Design review of the part built by this model. Coordinates are the model's own, in mm. A direction names the side the tool comes from. Coordinates: 2 decimals unless noted, no trailing zeros. Loops run counter-clockwise (first coordinate to the right, second up) from the corner with the lowest first, then second, coordinate; pieces in that order, holes last. Notation, with made-up numbers: M 56,13 L 96,13 A15 cw 96,40 Z; hole C 31.5,70.5 d9. An arc over 180 degrees is marked long. Answer as CSV lines item,"result". Start each with the question number.
from build123d import *

# Parameters (mm, degrees)
F2_DEPTH  = 5
F3_W      = 14.7
F3_H      = 25
F4_DEPTH  = 7.7
F6_DEPTH  = 5
F8_DEPTH  = 70
F10_DEPTH = 5
F12_DEPTH = 50.001


with BuildPart() as f2:
    # F1 (on Top) → F2 (new body)
    with BuildSketch(Plane.XY):
        Polygon((0, 50), (0, 0), (17.65, 0), (17.65, 25), (32.35, 25), (32.35, 0), (50, 0), (50, 50), align=None)
    extrude(amount=F2_DEPTH)

    # F3 (on face) → F4 (join)
    with BuildSketch(Plane.XY.offset(5)):
        with Locations((25, 37.5)):
            Rectangle(F3_W, F3_H)
    extrude(amount=F4_DEPTH)

    # F5 (on face) → F6 (join)
    with BuildSketch(Plane.XY.offset(12.7)):
        Polygon((0, 50), (0, 0), (17.65, 0), (17.65, 25), (32.35, 25), (32.35, 0), (50, 0), (50, 50), align=None)
    extrude(amount=F6_DEPTH)

    # F7 (on face) → F8 (join)
    with BuildSketch(Plane.XY.offset(17.7)):
        with BuildLine():
            Line((32.35, 25), (32.35, 1.104865))
            ThreePointArc((32.35, 1.104865), (25, 50), (17.65, 1.104865))
            Line((17.65, 1.104865), (17.65, 25))
            Line((17.65, 25), (32.35, 25))
        make_face()
    extrude(amount=F8_DEPTH)

    # F9 (on face) → F10 (join)
    with BuildSketch(Plane.XY.offset(87.7)):
        with BuildLine():
            Line((0, 35), (0, 25))
            Line((0, 25), (50, 25))
            Line((50, 25), (50, 35))
            ThreePointArc((50, 35), (25, 60), (0, 35))
        make_face()
    extrude(amount=F10_DEPTH)

    # F11 (on Right) → F12 (cut, through all)
    with BuildSketch(Plane.YZ):
        Polygon((1.104865, 17.7), (25, 87.7), (1.104865, 87.7), align=None)
    extrude(amount=F12_DEPTH, mode=Mode.SUBTRACT)


solid = f2.part
Item 1: For pin 1 (3 mm diameter, centred on y = 23, z = 47, fed in from -X) (3 decimals); pin 2 (3 mm diameter, centred on y = 47, z = 25.5, fed in from -X); pin 3 (10 mm diameter, centred on x = 45, y = 29, fed in from -Z); pin 4 (2.5 mm diameter, centred on y = 38.5, z = 7, fed in from -X), all flat-tipped, find the tip position at first contact; note any pin that passes through.
Item 2: Add section B-B (y = 9.5). Give the boundary of the cut face in (x, z), plus the area to 3 significant figures.
Item 3: For line 1 along Z through (x, y) = (13, 3); line 2 along Z through (x, y) = (7.5, 29); line 3 along Y through (x, z) = (38.5, 4.5), list the stretches that pass through material, from the lowest coordinate up. Write a range as from..to.
Item 4: Add section C-C (x = 30). Give the boundary of the cut face in (y, z), plus the area to 3 significant figures.
Item 5: Add section A-A (x = 9). Give the boundary of the cut face in (y, z), plus the area to 3 significant figures.
Item 6: Mouldability with a two-part tool opening along X and no side actions: class faces 1 (the face through (9, 0, 15)), 2 (the face through (50, 25, 2)), 3 (the face through (17.65, 12, 2)) as released by +X, released by -X, zero draft, split by the parting line, or undercut.
Item 7: For faces 4 (the face through (41, 25, 5)), 5 (the face through (44, 45, 17.7)), 6 (the face through (32.35, 13, 2)), list the 3-axis set-ups (+Z, -Z, +X, -X, +Y, -Y) from which the entire face can be reached by the end or side of a thin tool; tool diameter is ignored.
Response:
1,pin 1,"x = 0.005"
1,pin 2,"x = 10.69"
1,pin 3,"z = 0"
1,pin 4,"x = 17.65"
2,outline,"M 0,0 L 17.65,0 L 17.65,5 L 0,5 Z; M 0,12.7 L 17.65,12.7 L 17.65,42.29 L 5.38,42.29 L 5.38,17.7 L 0,17.7 Z; M 32.35,0 L 50,0 L 50,5 L 32.35,5 Z; M 32.35,12.7 L 50,12.7 L 50,17.7 L 44.62,17.7 L 44.62,42.29 L 32.35,42.29 Z"
2,area,"956 mm²"
3,line 1,"0..5, 12.7..17.7"
3,line 2,"0..5, 12.7..92.7"
3,line 3,"0..50"
4,outline,"M 25,0 L 50,0 L 50,17.7 L 49.49,17.7 L 49.49,87.7 L 59.49,87.7 L 59.49,92.7 L 25,92.7 Z"
4,area,"2,330 mm²"
5,outline,"M 0,0 L 50,0 L 50,5 L 0,5 Z; M 0,12.7 L 50,12.7 L 50,17.7 L 44.21,17.7 L 44.21,87.7 L 54.21,87.7 L 54.21,92.7 L 25,92.7 L 25,87.7 L 5.79,31.43 L 5.79,17.7 L 0,17.7 Z"
5,area,"2,790 mm²"
6,face 1,"zero draft"
6,face 2,"released by +X"
6,face 3,"undercut"
7,face 4,"+X, +Y, -Y"
7,face 5,"+X, +Y"
7,face 6,"+Z, -Z, -Y"
